Read the model definition and answer for the solid it produces. Units are mm, in the model's axes. Round coordinates to 2 decimals unless told otherwise and drop trailing zeros.
from build123d import *

# Parameters (mm, degrees)
SKETCH1_R               = 4.25
BOSS_EXTRUDE1_DEPTH     = 2
CUT_EXTRUDE1_DEPTH      = 253.36927309
CUT_EXTRUDE1_DEPTH_BACK = 253.36927309
SKETCH2_W               = 130
SKETCH2_H               = 36
SKETCH5_W               = 2
SKETCH5_H               = 40
SKETCH5_W_2             = 40
SKETCH5_H_2             = 2
BOSS_EXTRUDE2_DEPTH     = 2


with BuildPart() as part:
    # Sketch1 → Boss-Extrude1 (new body)
    with BuildSketch(Plane(origin=(0, 0, 0), x_dir=(1, 0, 0), z_dir=(0, 1, 0))):
        Polygon((64, -157.5), (162, -157.5), (162, 157.5), (-162, 157.5), (-162, -157.5), (-66, -157.5), (-66, -193.5), (64, -193.5), align=None)
        with Locations(Location((-51, -175.5, 0), (0, 0, 270))):
            Circle(SKETCH1_R, mode=Mode.SUBTRACT)
        with Locations(Location((49, -175.5, 0), (0, 0, 270))):
            Circle(SKETCH1_R, mode=Mode.SUBTRACT)
    extrude(amount=BOSS_EXTRUDE1_DEPTH)

    # Sketch2 → Cut-Extrude1 (cut, two sides: drawn at the far end of the back side and taken through both)
    with BuildSketch(Plane(origin=(0, 2, 0), x_dir=(1, 0, 0), z_dir=(0, 1, 0)).offset(-CUT_EXTRUDE1_DEPTH_BACK)):
        with Locations((-1, -175.5)):
            Rectangle(SKETCH2_W, SKETCH2_H)
    extrude(amount=CUT_EXTRUDE1_DEPTH + CUT_EXTRUDE1_DEPTH_BACK, mode=Mode.SUBTRACT)

    # Sketch5 → Boss-Extrude2 (add)
    with BuildSketch(Plane.XZ):
        with Locations((-163, 107.5)):
            Rectangle(SKETCH5_W, SKETCH5_H)
        with Locations((-163, 37.5)):
            Rectangle(SKETCH5_W, SKETCH5_H)
        with Locations((-112, 158.5)):
            Rectangle(SKETCH5_W_2, SKETCH5_H_2)
        with Locations((-42, 158.5)):
            Rectangle(SKETCH5_W_2, SKETCH5_H_2)
        with Locations((-163, -107.5)):
            Rectangle(SKETCH5_W, SKETCH5_H)
        with Locations((-163, -37.5)):
            Rectangle(SKETCH5_W, SKETCH5_H)
        with Locations((-112, -158.5)):
            Rectangle(SKETCH5_W_2, SKETCH5_H_2)
        with Locations((-42, -158.5)):
            Rectangle(SKETCH5_W_2, SKETCH5_H_2)
        with Locations((42, -158.5)):
            Rectangle(SKETCH5_W_2, SKETCH5_H_2)
        with Locations((112, -158.5)):
            Rectangle(SKETCH5_W_2, SKETCH5_H_2)
        with Locations((163, -37.5)):
            Rectangle(SKETCH5_W, SKETCH5_H)
        with Locations((163, -107.5)):
            Rectangle(SKETCH5_W, SKETCH5_H)
        with Locations((42, 158.5)):
            Rectangle(SKETCH5_W_2, SKETCH5_H_2)
        with Locations((112, 158.5)):
            Rectangle(SKETCH5_W_2, SKETCH5_H_2)
        with Locations((163, 37.5)):
            Rectangle(SKETCH5_W, SKETCH5_H)
        with Locations((163, 107.5)):
            Rectangle(SKETCH5_W, SKETCH5_H)
    extrude(amount=-BOSS_EXTRUDE2_DEPTH)


solid = part.part
Q1. Flat-ended cylindrical pins translate along their axes: pin 1 Ø0.6 at (x, y) = (163, 1) entering from +Z; pin 2 Ø0.6 at (y, z) = (0.5, -159) entering from +X; pin 3 Ø0.6 at (x, y) = (-163, 1.5) entering from -Z. Find the tip coordinate at first contact, or state that the pin passes through.
Verdict:
pin 1: stops at z = 127.5
pin 2: stops at x = 132
pin 3: stops at z = -127.5
Q2. Straight lines are drawn through the part: probe 1 along X at (y, z) = (1.45, 0); probe 2 along Z at (x, y) = (134, 1.8). For each, find the intervals that lie inside material, in ascending order.
Verdict:
probe 1: x = -162 to 162
probe 2: z = -157.5 to 157.5
Q3. Determine the mould class of faces 1 (the flat face through (-2, 2, -2)), 2 (the flat face through (-2, 0, -2)) for opening direction Y: pulls with the +Y half, pulls with the -Y half, needs draft (parallel to the pull), parting line crosses it, or undercut.
Verdict:
face 1: pulls with the +Y half
face 2: pulls with the -Y half
